from build123d import *

# Parameters (mm, degrees)
F0_W     = 76.2029737234
F0_H     = 50.7892221212
F1_DEPTH = 76.2
F2_DEPTH = 76.2
F3_W     = 25.3895288229
F3_H     = 12.7094006166
F4_DEPTH = 169.164


with BuildPart() as f1:
    # F0 (on Right) → F1 (new body)
    with BuildSketch(Plane.YZ):
        Rectangle(F0_W, F0_H)
    extrude(amount=F1_DEPTH)

    # F2 (add): a face of the model
    f2_faces = [f1.faces().sort_by_distance(p)[0] for p in [
        (0, 0, 0),
    ]]
    extrude(f2_faces, amount=F2_DEPTH)

    # F3 (on face) → F4 (cut)
    with BuildSketch(Plane(origin=(0, 38.1014868617, 0), x_dir=(-1, 0, 0), z_dir=(0, 1, 0))):
        Polygon((-50.7960021496, -12.6930763945), (-38.0911789834, -25.3946110606), (38.0879864097, -25.3946110606), (50.7873259485, -12.705120258), align=None)
        Polygon((76.2, 25.3946110606), (50.8108735085, 25.3946110606), (38.1050296128, 12.685210444), (50.8108735085, 12.685210444), (76.2, 12.685210444), align=None)
        Polygon((-50.8104711771, 25.3946110606), (-50.8104711771, 12.685210444), (-38.1180383265, 12.685210444), align=None)
        with Locations((-63.5052355886, 19.0399107523)):
            Rectangle(F3_W, F3_H)
    extrude(amount=-F4_DEPTH, mode=Mode.SUBTRACT)


solid = f1.part
Could you check a few things on this model? Use its own coordinates, in mm. A direction names the side the tool comes from. Round coordinates to 2 decimals unless told otherwise and drop trailing zeros. Order: outer loops, then holes, each group sorted by start corner. A loop starts at its lowest first (then second) coordinate and runs counter-clockwise, first axis right, second up.
Q1. Please list where these lines run through material, in increasing order: probe 1 along Z at (x, y) = (12, 11); probe 2 along Z at (x, y) = (57, 33.5); probe 3 along X at (y, z) = (-13, -14.5).
Geometry says:
probe 1: z = -12.7 to 25.39
probe 2: z = -25.39 to 12.69
probe 3: x = -76.2 to -48.99, 48.99 to 76.2
Q2. Imagine slicing it at D-D, the plane x = 59. List the corners of the cut face in (y, z) for me, then the cut area to 3 significant figures.
Geometry says:
outline: (-38.1, -25.39) - (38.1, -25.39) - (38.1, 12.69) - (-38.1, 12.69) - close
area: 2,900 mm2
Q3. Imagine slicing it at A-A, the plane z = -20.5. List the corners of the cut face in (x, y) for me, then the cut area to 3 significant figures.
Geometry says:
outline: (-76.2, -38.1) - (-42.99, -38.1) - (-42.99, 38.1) - (-76.2, 38.1) - close; (42.99, -38.1) - (76.2, -38.1) - (76.2, 38.1) - (42.99, 38.1) - close
area: 5,060 mm2
Q4. I'm going to push flat-ended pins straight in: P1, Ø3, axis at y = -2, z = 15.5, coming from the +X side; P2, Ø19, axis at x = 61.5, y = 16.5, coming from the +Z side; P3, Ø5, axis at x = -43.5, z = -18.5, coming from the -Y side; P4, Ø1.5, axis at x = 16, y = -16.5, coming from the -Z side. Where does each tip first touch, or does it pass through?
Geometry says:
P1: stops at x = 42.43
P2: stops at z = 12.69
P3: stops at y = -38.1
P4: stops at z = -12.7
Q5. Imagine slicing it at B-B, the plane y = -0.5. List the corners of the cut face in (x, z) for me.
Geometry says:
outline: (-76.2, -25.39) - (-38.09, -25.39) - (-50.79, -12.71) - (50.8, -12.69) - (38.09, -25.39) - (76.2, -25.39) - (76.2, 12.69) - (38.12, 12.69) - (50.81, 25.39) - (-50.81, 25.39) - (-38.11, 12.69) - (-76.2, 12.69) - close
Q6. Imagine slicing it at C-C, the plane x = -47. List the corners of the cut face in (y, z) for me.
Geometry says:
outline: (-38.1, -25.39) - (38.1, -25.39) - (38.1, -16.49) - (-38.1, -16.49) - close; (-38.1, -12.7) - (38.1, -12.7) - (38.1, 12.69) - (-38.1, 12.69) - close; (-38.1, 21.58) - (38.1, 21.58) - (38.1, 25.39) - (-38.1, 25.39) - close
Q7. Thinking about a two-plate mould opening in X: for faces 1 (the face through (-57, 1, 12.685)), 2 (the face through (-44.35, 0.53, -19.14)), 3 (the face through (-44.55, 0.53, 19.13)), 4 (the face through (76.2, -1, -6)), which applies, released by +X, released by -X, zero draft, split by the parting line, or undercut?
Geometry says:
face 1: zero draft
face 2: undercut
face 3: released by -X
face 4: released by +X
Q8. Which directions (+Z, -Z, +X, -X, +Y, -Y) give clear straight access to the entire face, cutting with the end or side of a thin tool? Please do faces 5 (the face through (44.375, 0.533, 18.951)), 6 (the face through (57, -1, -25.395)).
Geometry says:
face 5: +X, +Y, -Y
face 6: -Z, +X, -X, +Y, -Y
